Geometry: final body of the model. Coordinates: model frame, mm. A direction names the side the tool comes from. Round coordinates to 2 decimals unless told otherwise and drop trailing zeros. Write each loop counter-clockwise with the first axis right and the second up, starting at its lowest first coordinate (ties: lowest second). Pieces come first, ordered by that corner, then holes. Notation, with made-up numbers: M 77,43 L 108,43 A20 cw 108,77 Z; hole C 58.25,-17 d3. An arc over 180 degrees is marked long. Use one line per item in the form item = value. Start each with the question number.
Item 1: Section query B-B (x = 211.5). Return loops of the section in (y, z).
Item 2: Pin query (flat end, axial travel): pin 1 Ø8 at (x, y) = (30, 45) entering from -Z; pin 2 Ø2.5 at (y, z) = (60, 3.5) entering from +X; pin 3 Ø4 at (y, z) = (48.5, 1) entering from -X; pin 4 Ø3.5 at (x, z) = (297, 4) entering from +Y. Return the tip coordinate at first contact, or that it passes through.
Item 3: Section query D-D (x = 133). Return loops of the section in (y, z), and give its area (3 significant figures).
Item 4: Reachability of faces 1 (the flat face through (264, 0, 4)), 2 (the flat face through (264, 57, 4)), 3 (the flat face through (168, 29, 0)), 4 (the flat face through (194.247, 23, 4)) from +Z, -Z, +X, -X, +Y, -Y: full face, straight path, thin tool, end or side. Return the list, or none.
Item 5: Section query A-A (x = 310). Return loops of the section in (y, z).
Item 6: Ray query, probe 1 along Z at (x, y) = (43, 51.25); probe 2 along Y at (x, z) = (89, 4.25); probe 3 along Y at (x, z) = (243, 3.25). Return the intervals inside material, ascending.
Item 7: Pull-direction query (Y, two-part tool) for faces 5 (the flat face through (76, 0, 3)), 6 (the flat face through (253, 47, 4)), 7 (the flat face through (79, 57, 3)), 8 (the flat face through (340, 28, 7)); classes: pulls with the +Y half, pulls with the -Y half, needs draft (parallel to the pull), parting line crosses it, or undercut.
Item 8: Section query C-C (x = 170). Return loops of the section in (y, z), and give its area (3 significant figures).
from build123d import *

# Parameters (mm, degrees)
RESSALTO_EXTRUS_O1_DEPTH                    = 8
BROCA_DE_ROSQUEAR_PARA_TARRAXA_DE_M82_D     = 6.8
ESBO_O8_W                                   = 28
ESBO_O8_H                                   = 57
RESSALTO_EXTRUS_O2_DEPTH                    = 1
BROCA_DE_ROSQUEAR_PARA_TARRAXA_DE_M61_D     = 5
BROCA_DE_ROSQUEAR_PARA_TARRAXA_DE_M61_DEPTH = 15
BROCA_DE_ROSQUEAR_PARA_TARRAXA_DE_M61_TIP   = 1.502151548
BROCA_DE_ROSQUEAR_PARA_TARRAXA_DE_M62_D     = 5
BROCA_DE_ROSQUEAR_PARA_TARRAXA_DE_M62_DEPTH = 15
BROCA_DE_ROSQUEAR_PARA_TARRAXA_DE_M62_TIP   = 1.502151548
CHANFRO2_SIZE                               = 7
CHANFRO3_SIZE                               = 7
CORTE_EXTRUS_O1_DEPTH                       = 10
FILETE1_R                                   = 2
BROCA_DE_ROSQUEAR_PARA_TARRAXA_DE_M51_D     = 4.2
BROCA_DE_ROSQUEAR_PARA_TARRAXA_DE_M51_DEPTH = 15
BROCA_DE_ROSQUEAR_PARA_TARRAXA_DE_M51_TIP   = 1.2618073
BROCA_DE_ROSQUEAR_PARA_TARRAXA_DE_M52_D     = 4.2
BROCA_DE_ROSQUEAR_PARA_TARRAXA_DE_M52_DEPTH = 15
BROCA_DE_ROSQUEAR_PARA_TARRAXA_DE_M52_TIP   = 1.2618073
FILETE2_R                                   = 2


with BuildPart() as part:
    # Esboço1 → Ressalto-extrusão1 (new body)
    with BuildSketch(Plane.XY):
        Polygon((185, 57), (185, 62), (155, 62), (155, 57), (0, 57), (0, 0), (155, 0), (155, -5), (185, -5), (185, 0), (340, 0), (340, 57), align=None)
    extrude(amount=RESSALTO_EXTRUS_O1_DEPTH)

    # Broca de rosquear para tarraxa de M82 (through all)
    with Locations(Plane.XY.offset(8)):
        with Locations((30, 45), (30, 12), (170, 45), (170, 12), (310, 45), (310, 12)):
            Hole(BROCA_DE_ROSQUEAR_PARA_TARRAXA_DE_M82_D / 2)

    # Esboço8 → Ressalto-extrusão2 (add)
    with BuildSketch(Plane(origin=(0, 0, 0), x_dir=(-1, 0, 0), z_dir=(0, 0, -1))):
        with Locations((-326, 28.5)):
            Rectangle(ESBO_O8_W, ESBO_O8_H)
        with Locations((-14, 28.5)):
            Rectangle(ESBO_O8_W, ESBO_O8_H)
    extrude(amount=RESSALTO_EXTRUS_O2_DEPTH)

    # Broca de rosquear para tarraxa de M61
    with Locations(Plane(origin=(340, 0, 0), x_dir=(0, 0, -1), z_dir=(1, 0, 0))):
        with Locations((-3, 46), (-3.5, 28.5), (-3.5, 11)):
            Hole(BROCA_DE_ROSQUEAR_PARA_TARRAXA_DE_M61_D / 2, depth=BROCA_DE_ROSQUEAR_PARA_TARRAXA_DE_M61_DEPTH)
            with Locations((0, 0, -(BROCA_DE_ROSQUEAR_PARA_TARRAXA_DE_M61_DEPTH + BROCA_DE_ROSQUEAR_PARA_TARRAXA_DE_M61_TIP / 2))):  # 118° drill point
                Cone(0, BROCA_DE_ROSQUEAR_PARA_TARRAXA_DE_M61_D / 2, BROCA_DE_ROSQUEAR_PARA_TARRAXA_DE_M61_TIP, mode=Mode.SUBTRACT)

    # Broca de rosquear para tarraxa de M62
    with Locations(Plane.ZY):
        with Locations((3, 46), (3, 11), (3, 28.5)):
            Hole(BROCA_DE_ROSQUEAR_PARA_TARRAXA_DE_M62_D / 2, depth=BROCA_DE_ROSQUEAR_PARA_TARRAXA_DE_M62_DEPTH)
            with Locations((0, 0, -(BROCA_DE_ROSQUEAR_PARA_TARRAXA_DE_M62_DEPTH + BROCA_DE_ROSQUEAR_PARA_TARRAXA_DE_M62_TIP / 2))):  # 118° drill point
                Cone(0, BROCA_DE_ROSQUEAR_PARA_TARRAXA_DE_M62_D / 2, BROCA_DE_ROSQUEAR_PARA_TARRAXA_DE_M62_TIP, mode=Mode.SUBTRACT)

    # Chanfro2
    # the kernel refuses this chamfer: 7 mm, written as the material it takes off along each edge
    with BuildSketch(Plane(origin=(28, -18.001780916, -1), x_dir=(0.02749587661058661, 0, 0.9996219169112968), z_dir=(0, 1, 0))) as chanfro2_piece_1_section:
        Polygon((CHANFRO2_SIZE * 0.999621916911, -CHANFRO2_SIZE * 0.0274958766106), (-CHANFRO2_SIZE * 0.0274958766106, -CHANFRO2_SIZE * 0.999621916911), (0, 0), align=None)
    chanfro2_piece_1 = extrude(amount=93.003561832, mode=Mode.PRIVATE)
    chanfro2_piece_1 = split(chanfro2_piece_1, bisect_by=Plane(origin=(24.64888361, 28.5, 0), z_dir=(0, 0, -1)), keep=Keep.TOP, mode=Mode.PRIVATE)
    add(chanfro2_piece_1, mode=Mode.SUBTRACT)

    # Chanfro3
    # the kernel refuses this chamfer: 7 mm, written as the material it takes off along each edge
    with BuildSketch(Plane(origin=(312, -18.001780916, -1), x_dir=(-0.027495876610590064, 0, 0.9996219169112966), z_dir=(0, 1, 0))) as chanfro3_piece_1_section:
        Polygon((CHANFRO3_SIZE * 0.999621916911, CHANFRO3_SIZE * 0.0274958766106), (-CHANFRO3_SIZE * 0.0274958766106, CHANFRO3_SIZE * 0.999621916911), (0, 0), align=None)
    chanfro3_piece_1 = extrude(amount=93.003561832, mode=Mode.PRIVATE)
    chanfro3_piece_1 = split(chanfro3_piece_1, bisect_by=Plane(origin=(315.35111639, 28.5, 0), z_dir=(0, 0, -1)), keep=Keep.TOP, mode=Mode.PRIVATE)
    add(chanfro3_piece_1, mode=Mode.SUBTRACT)

    # Esboço10 → Corte-extrusão1 (cut)
    with BuildSketch(Plane(origin=(0, 0, 0), x_dir=(-1, 0, 0), z_dir=(0, 0, -1))):
        Polygon((-285.753328204, 47), (-210.753328204, 47), (-285.753328204, 20), align=None)
        Polygon((-269.246671796, 10), (-194.246671796, 37), (-194.246671796, 10), align=None)
        Polygon((-145.753328204, 10), (-70.753328204, 10), (-145.753328204, 37), align=None)
        Polygon((-54.246671796, 20), (-54.246671796, 47), (-129.246671796, 47), align=None)
    extrude(amount=-CORTE_EXTRUS_O1_DEPTH, mode=Mode.SUBTRACT)

    # Filete1
    filete1_edges = [part.edges().sort_by_distance(p)[0] for p in [
        (194.246671796, 10, 4),
        (269.246671796, 10, 4),
        (194.246671796, 37, 4),
        (285.753328204, 20, 4),
        (285.753328204, 47, 4),
        (210.753328204, 47, 4),
    ]]
    fillet(filete1_edges, radius=FILETE1_R)

    # Broca de rosquear para tarraxa de M51
    with Locations(Plane(origin=(0, 57, 0), x_dir=(1, 0, 0), z_dir=(0, 1, 0))):
        with Locations((43, -4), (142, -4), (198, -4), (297, -4)):
            Hole(BROCA_DE_ROSQUEAR_PARA_TARRAXA_DE_M51_D / 2, depth=BROCA_DE_ROSQUEAR_PARA_TARRAXA_DE_M51_DEPTH)
            with Locations((0, 0, -(BROCA_DE_ROSQUEAR_PARA_TARRAXA_DE_M51_DEPTH + BROCA_DE_ROSQUEAR_PARA_TARRAXA_DE_M51_TIP / 2))):  # 118° drill point
                Cone(0, BROCA_DE_ROSQUEAR_PARA_TARRAXA_DE_M51_D / 2, BROCA_DE_ROSQUEAR_PARA_TARRAXA_DE_M51_TIP, mode=Mode.SUBTRACT)

    # Broca de rosquear para tarraxa de M52
    with Locations(Plane(origin=(0, 0, 0), x_dir=(-1, 0, 0), z_dir=(0, -1, 0))):
        with Locations((-150, -4), (-190, -4), (-297, -4), (-43, -4), (-272, -4), (-68, -4)):
            Hole(BROCA_DE_ROSQUEAR_PARA_TARRAXA_DE_M52_D / 2, depth=BROCA_DE_ROSQUEAR_PARA_TARRAXA_DE_M52_DEPTH)
            with Locations((0, 0, -(BROCA_DE_ROSQUEAR_PARA_TARRAXA_DE_M52_DEPTH + BROCA_DE_ROSQUEAR_PARA_TARRAXA_DE_M52_TIP / 2))):  # 118° drill point
                Cone(0, BROCA_DE_ROSQUEAR_PARA_TARRAXA_DE_M52_D / 2, BROCA_DE_ROSQUEAR_PARA_TARRAXA_DE_M52_TIP, mode=Mode.SUBTRACT)

    # Filete2
    filete2_edges = [part.edges().sort_by_distance(p)[0] for p in [
        (145.753328204, 10, 4),
        (145.753328204, 37, 4),
        (70.753328204, 10, 4),
        (54.246671796, 20, 4),
        (129.246671796, 47, 4),
        (54.246671796, 47, 4),
    ]]
    fillet(filete2_edges, radius=FILETE2_R)


solid = part.part
Working result:
q1.outline = M 0,0 L 10,0 L 10,8 L 0,8 Z; M 30.79,0 L 57,0 L 57,8 L 30.79,8 Z
q2.pin_1 = 0
q2.pin_2 = 185
q2.pin_3 = 0
q2.pin_4 = 41.79
q3.outline = M 0,0 L 10,0 L 10,8 L 0,8 Z; M 32.41,0 L 57,0 L 57,8 L 32.41,8 Z
q3.area = 277 mm²
q4.face_1 = +Z, -Z, +X, -Y
q4.face_2 = +Z, -Z, +X, +Y
q4.face_3 = -Z, +Y, -Y
q4.face_4 = +Z, -Z
q5.outline = M 0,0 L 8.6,0 L 8.6,8 L 0,8 Z; M 15.4,0 L 41.6,0 L 41.6,8 L 15.4,8 Z; M 48.4,0 L 57,0 L 57,8 L 48.4,8 Z
q6.probe_1 = 0 to 1.9, 6.1 to 8
q6.probe_2 = 0 to 10, 16.57 to 32.51, 47 to 57
q6.probe_3 = 0 to 10, 19.45 to 35.39, 47 to 57
q7.face_5 = pulls with the -Y half
q7.face_6 = undercut
q7.face_7 = pulls with the +Y half
q7.face_8 = needs draft
q8.outline = M -5,0 L 8.6,0 L 8.6,8 L -5,8 Z; M 15.4,0 L 41.6,0 L 41.6,8 L 15.4,8 Z; M 48.4,0 L 62,0 L 62,8 L 48.4,8 Z
q8.area = 427 mm²
